```python
from build123d import *

# Parameters (mm, degrees)
SKETCH2_R           = 15.875
BOSS_EXTRUDE1_DEPTH = 53.34
SKETCH3_R           = 4.3053
BOSS_EXTRUDE2_DEPTH = 24.13
SKETCH4_R           = 3.175
BOSS_EXTRUDE3_DEPTH = 16.51
SKETCH5_OUTSIDE_W   = 51.704
SKETCH5_OUTSIDE_H   = 52.339
SKETCH5_OUTSIDE_R   = 14.605
CUT_EXTRUDE1_DEPTH  = 16.51


with BuildPart() as part:
    # Sketch2 → Boss-Extrude1 (new body)
    with BuildSketch(Plane.XY):
        Circle(SKETCH2_R)
    extrude(amount=BOSS_EXTRUDE1_DEPTH)

    # Sketch3 → Boss-Extrude2 (add)
    with BuildSketch(Plane(origin=(0, 0, 0), x_dir=(-1, 0, 0), z_dir=(0, 0, -1))):
        Polygon((8.248891971, 0), (4.124445986, 7.14375), (-4.124445986, 7.14375), (-8.248891971, 0), (-4.124445986, -7.14375), (4.124445986, -7.14375), align=None)
        Circle(SKETCH3_R, mode=Mode.SUBTRACT)
    extrude(amount=BOSS_EXTRUDE2_DEPTH)

    # Sketch4 → Boss-Extrude3 (add)
    with BuildSketch(Plane(origin=(0, 0, 0), x_dir=(1, 0, 0), z_dir=(0, 1, 0))):
        with Locations(Location((1.475733324, -26.436178991, 0), (0, 0, 270))):
            Circle(SKETCH4_R)
    extrude(amount=-BOSS_EXTRUDE3_DEPTH)

    # Sketch5 outside → Cut-Extrude1 (cut)
    with BuildSketch(Plane.XY.offset(53.34)):
        with Locations((0, -0.3175)):
            Rectangle(SKETCH5_OUTSIDE_W, SKETCH5_OUTSIDE_H)
        Circle(SKETCH5_OUTSIDE_R, mode=Mode.SUBTRACT)
    extrude(amount=-CUT_EXTRUDE1_DEPTH, mode=Mode.SUBTRACT)


solid = part.part
```
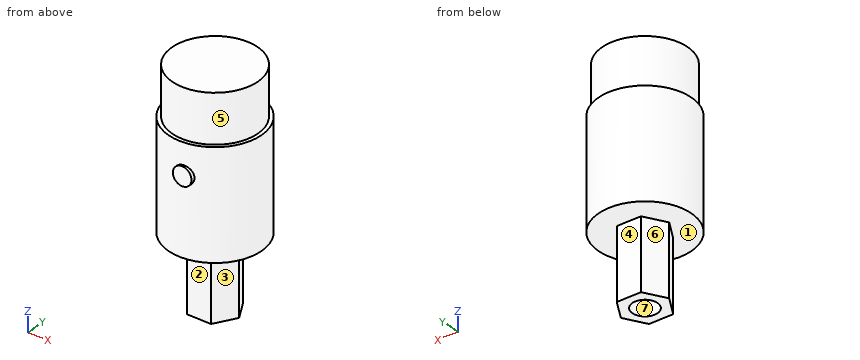
The listing builds one solid part. Answer for the finished solid, in the listing's coordinates (mm). Face numbers are marked on the shaded views. A direction names the side the tool comes from. Coordinates: 2 decimals unless noted, no trailing zeros. Write each loop counter-clockwise with the first axis right and the second up, starting at its lowest first coordinate (ties: lowest second). Pieces come first, ordered by that corner, then holes. Notation, with made-up numbers: (44.5, -7.5) - (94.5, -7.5) arc R25 cw to (94.5, 7.5) - close; hole circle Ø6 at (21.25, 76.5). An arc over 180 degrees is marked (long way). Return JSON: item names as keys, results as strings. Group by question number.
1. A cutting plane is placed at A-A, the plane z = -17. Determine the outline of the cut face in (x, y).
2. Determine the mould class of the marked faces 4, 5, 6 and 7 for opening direction X: released by +X, released by -X, zero draft, split by the parting line, or undercut.
3. Which of the six approach directions +Z, -Z, +X, -X, +Y, -Y give full straight-line access (tool end or side, diameter ignored) to the marked faces 1, 2 and 3?
4. A cutting plane is placed at C-C, the plane y = -8. Determine the outline of the cut face in (x, z).
5. Given pin 1 (2.5 mm diameter, centred on x = 0, z = -10, fed in from +Y); pin 2 (6.5 mm diameter, centred on x = -2, z = -17.5, fed in from -Y); pin 3 (1 mm diameter, centred on y = -2.5, z = 32, fed in from -X), each flat-ended and moving along its own axis, determine where each tip first touches the part or whether it passes through.
6. A cutting plane is placed at D-D, the plane y = 11. Determine the outline of the cut face in (x, z).
7. Straight lines are drawn through the part: L1, parallel to Y at x = 0, z = -8.75; L2, parallel to Z at x = 4, y = -9; L3, parallel to Y at x = -1, z = -6. For each, find the intervals that lie inside material, in ascending order.
8. A cutting plane is placed at B-B, the plane x = -6.5. Determine the outline of the cut face in (y, z).
Ans:
{
 "1": {"outline": "(-8.25, 0) - (-4.12, -7.14) - (4.12, -7.14) - (8.25, 0) - (4.12, 7.14) - (-4.12, 7.14) - close; hole circle Ø8.61 at (0, 0)"},
 "2": {"face 4": "zero draft", "face 5": "split by the parting line", "face 6": "released by -X", "face 7": "undercut"},
 "3": {"face 1": "-Z", "face 2": "-Z, +X, -X, -Y", "face 3": "-Z, +X, -Y"},
 "4": {"outline": "(-13.71, 0) - (13.71, 0) - (13.71, 36.83) - (12.22, 36.83) - (12.22, 53.34) - (-12.22, 53.34) - (-12.22, 36.83) - (-13.71, 36.83) - close"},
 "5": {"pin 1": "y = 7.14", "pin 2": "y = -7.14", "pin 3": "x = -15.75"},
 "6": {"outline": "(-11.45, 0) - (11.45, 0) - (11.45, 36.83) - (9.61, 36.83) - (9.61, 53.34) - (-9.61, 53.34) - (-9.61, 36.83) - (-11.45, 36.83) - close"},
 "7": {"L1": "-7.14 to -4.31, 4.31 to 7.14", "L2": "0 to 53.34", "L3": "-7.14 to -4.19, 4.19 to 7.14"},
 "8": {"outline": "(-14.48, 0) - (-3.03, 0) - (-3.03, -24.13) - (3.03, -24.13) - (3.03, 0) - (14.48, 0) - (14.48, 36.83) - (13.08, 36.83) - (13.08, 53.34) - (-13.08, 53.34) - (-13.08, 36.83) - (-14.48, 36.83) - close"}
}
